```python
from build123d import *

# Parameters (mm, degrees)
CUT_EXTRUDE2_DEPTH  = 7
SKETCH2_R           = 13
CUT_EXTRUDE1_DEPTH  = 4.5
SKETCH5_R           = 11.4
SKETCH5_R_2         = 8.198373822
BOSS_EXTRUDE2_DEPTH = 0.8
SKETCH6_R           = 13
SKETCH6_R_2         = 12
CUT_EXTRUDE3_DEPTH  = 1.5


with BuildPart() as part:
    # Sketch1 → Revolve1 (revolve)
    with BuildSketch(Plane(origin=(0, 0, 0), x_dir=(1, 0, 0), z_dir=(0, 1, 0))):
        with BuildLine():
            Line((6.15, -14.25), (6.15, 0))
            Line((6.15, 0), (8, 0))
            ThreePointArc((8, 0), (11.807886553, -0.781598043), (15, -3))
            Line((15, -3), (15, -4.25))
            Line((15, -4.25), (11.4, -4.25))
            Line((11.4, -4.25), (11.4, -14.25))
            Line((11.4, -14.25), (6.15, -14.25))
        make_face()
    revolve(axis=Axis((0, 0, 0), (0, 0, 1)))

    # Sketch3 → Cut-Extrude2 (cut)
    with BuildSketch(Plane.XY.offset(14.25)):
        Polygon((0, -8.198373822), (7.1, -4.099186911), (7.1, 4.099186911), (0, 8.198373822), (-7.1, 4.099186911), (-7.1, -4.099186911), align=None)
    extrude(amount=-CUT_EXTRUDE2_DEPTH, mode=Mode.SUBTRACT)

    # Sketch2 → Cut-Extrude1 (cut)
    with BuildSketch(Plane.XY.offset(14.25)):
        Circle(SKETCH2_R)
    extrude(amount=-CUT_EXTRUDE1_DEPTH, mode=Mode.SUBTRACT)

    # Sketch5 → Boss-Extrude2 (add)
    with BuildSketch(Plane.XY.offset(9.75)):
        Circle(SKETCH5_R)
        Circle(SKETCH5_R_2, mode=Mode.SUBTRACT)
    extrude(amount=BOSS_EXTRUDE2_DEPTH)

    # Sketch6 → Cut-Extrude3 (cut)
    with BuildSketch(Plane.XY.offset(4.25)):
        Circle(SKETCH6_R)
        Circle(SKETCH6_R_2, mode=Mode.SUBTRACT)
    extrude(amount=-CUT_EXTRUDE3_DEPTH, mode=Mode.SUBTRACT)


solid = part.part
```
Check sheet for the modelled part. Datum: model origin and axes. Units: mm. A direction names the side the tool comes from. Round coordinates to 2 decimals unless told otherwise and drop trailing zeros. Loops run counter-clockwise (first coordinate to the right, second up) from the corner with the lowest first, then second, coordinate; pieces in that order, holes last. Notation, with made-up numbers: (72.5, -23) - (81.5, -23) arc R26 ccw to (81.5, 9) - close; hole circle Ø8 at (-11, -26.5). An arc over 180 degrees is marked (long way). Answer as a JSON object with one key per item and string values. Group by question number.
Q1. Gauge pin test, flat ends, axial feed: P1, Ø3, axis at y = -10.5, z = 8, coming from the -X side; P2, Ø2, axis at x = -12, y = 9.5, coming from the +Z side; P3, Ø3, axis at x = -10, z = 1, coming from the +Y side; P4, Ø7.5, axis at x = 0, y = 0, coming from the +Z side. Record the tip position at first contact, or that the pin passes through.
Q2. Sectioned sample at A-A, the plane z = 8.5. Enter the section's corners in (x, y).
Q3. Scan lines: line 1 along Y through (x, z) = (0, 3.8); line 2 along Y through (x, z) = (0, 10.3); line 3 along Z through (x, y) = (-3.5, -7). Record each from-to range of solid material in increasing order. Write a range as [from, to].
Q4. Set-up check for faces 4 (the face through (2, -6, 0)), 5 (the face through (2, -6, 7.25)): record each of +Z, -Z, +X, -X, +Y, -Y from which the full face is reachable in a straight line by a thin tool's end or side.
Q5. Mould release check, pull along X, two halves, no side actions. Record for faces 1 (the face through (-14.985, 0.66, 3.634)), 2 (the face through (7.1, 0, 9)), 3 (the face through (11, -4, 4.25)): released by +X, released by -X, zero draft, split by the parting line, or undercut.
Q6. Sectioned sample at B-B, the plane z = 6.25. Enter the section's corners in (x, y).
Solution:
{
 "1": {"P1": "stops at x = -7", "P2": "stops at z = 4.25", "P3": "stops at y = 10.85", "P4": "passes through"},
 "2": {"outline": "circle Ø22.8 at (0, 0); hole (-7.1, -4.1) - (0, -8.2) - (7.1, -4.1) - (7.1, 4.1) - (0, 8.2) - (-7.1, 4.1) - close"},
 "3": {"line 1": "y = [-15, -13], [-12, -6.15], [6.15, 12], [13, 15]", "line 2": "y = [-11.4, -8.2], [8.2, 11.4]", "line 3": "z = [0, 9.75]"},
 "4": {"face 4": "-Z, +X, -X, +Y, -Y", "face 5": "+Z"},
 "5": {"face 1": "split by the parting line", "face 2": "undercut", "face 3": "zero draft"},
 "6": {"outline": "circle Ø22.8 at (0, 0); hole circle Ø12.3 at (0, 0)"}
}
